Geometry check sheet. Reference: the model listing, model coordinates, mm. Face numbers are marked on the shaded views. A direction names the side the tool comes from. Round coordinates to 2 decimals unless told otherwise and drop trailing zeros. Order: outer loops, then holes, each group sorted by start corner. A loop starts at its lowest first (then second) coordinate and runs counter-clockwise, first axis right, second up. Notation, with made-up numbers: (60, 6) -> (110, 6) arc R24 cw to (110, 28) -> close; hole circle Ø10 at (69, 2.5). An arc over 180 degrees is marked (long way). Use a Markdown table: item, result. Add a question column.
Item 1: Gauge pin test, flat ends, axial feed: pin 1 Ø1 at (x, z) = (-2, 1) entering from -Y; pin 2 Ø1 at (x, z) = (2.5, 0) entering from +Y; pin 3 Ø3 at (x, y) = (-1.5, 2) entering from +Z. Record the tip position at first contact, or that the pin passes through.
Item 2: Sectioned sample at D-D, the plane x = -2.25. Record the cut outline in (y, z), and give its area (3 significant figures).
Item 3: Set-up check for the marked faces 4 and 5: record each of +Z, -Z, +X, -X, +Y, -Y from which the full face is reachable in a straight line by a thin tool's end or side.
Item 4: Material ranges on probe 1 along Y at (x, z) = (0, -1.95); probe 2 along Y at (x, z) = (0, 0.1); probe 3 along Z at (x, y) = (2.25, -2), recorded low to high. Write a range as [from, to].
Item 5: Sectioned sample at A-A, the plane x = 0. Record the cut outline in (y, z), and give its area (3 significant figures).
Item 6: Sectioned sample at C-C, the plane z = 0.25. Record the cut outline in (x, y), and give its area (3 significant figures).
Item 7: Mould release check, pull along X, two halves, no side actions. Record for the marked faces 1, 2 and 3: pulls with the +X half, pulls with the -X half, needs draft (parallel to the pull), parting line crosses it, or undercut.
Autodesk Inventor part; units mm, degrees
ref_plane "YZ Plane" through (0, 0, 0) normal (1, 0, 0) x (0, 1, 0)
ref_plane "XZ Plane" through (0, 0, 0) normal (0, 1, 0) x (-1, 0, 0)
ref_plane "XY Plane" through (0, 0, 0) normal (0, 0, 1) x (1, 0, 0)
sketch "スケッチ1" plane through (0, 0, 0) normal (0, 0, 1) x (1, 0, 0)
  circle A0 centre (0, 0) radius 1.5
  circle A1 centre (0, 0) radius 4
  circle A2 centre (0, 0) radius 2
  circle A3 centre (0, 0) radius 3.5
  dimension "d0" = 3
  dimension "d1" = 8
  dimension "d2" = 4
  dimension "d3" = 0.5
extrude "押し出し1" add sketch "スケッチ1" along normal blind 2 contours A1 | A2 | A3
extrude "押し出し2" cut sketch "スケッチ1" against normal blind 0.1 from surface at 2 contours A3
mirror "ミラー1" about plane through (0, 0, 0) normal (0, 0, -1) of "押し出し1", "押し出し2"
properties part number "693ZZ" material "ステンレス鋼"
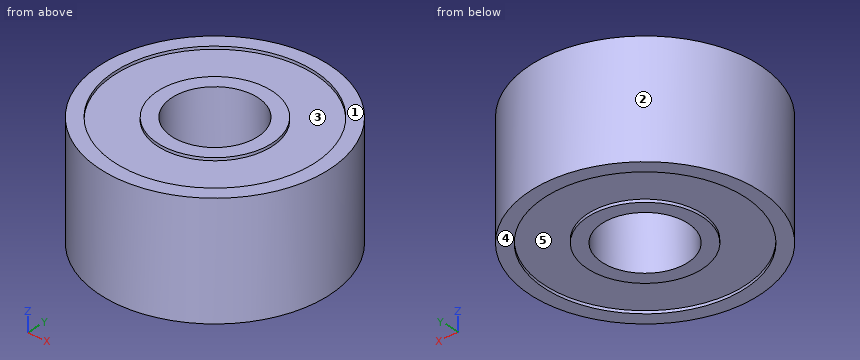
Found:
| question | item | result |
|---|---|---|
| 1 | pin 1 | stops at y = -3.71 |
| 1 | pin 2 | stops at y = 3.46 |
| 1 | pin 3 | stops at z = 2 |
| 2 | outline | (-3.31, -2) -> (-2.68, -2) -> (-2.68, -1.9) -> (2.68, -1.9) -> (2.68, -2) -> (3.31, -2) -> (3.31, 2) -> (2.68, 2) -> (2.68, 1.9) -> (-2.68, 1.9) -> (-2.68, 2) -> (-3.31, 2) -> close |
| 2 | area | 25.4 mm2 |
| 3 | face 4 | -Z, +X, -X, +Y, -Y |
| 3 | face 5 | -Z |
| 4 | probe 1 | y = [-4, -3.5], [-2, -1.5], [1.5, 2], [3.5, 4] |
| 4 | probe 2 | y = [-4, -1.5], [1.5, 4] |
| 4 | probe 3 | z = [-1.9, 1.9] |
| 5 | outline | (-4, -2) -> (-3.5, -2) -> (-3.5, -1.9) -> (-2, -1.9) -> (-2, -2) -> (-1.5, -2) -> (-1.5, 2) -> (-2, 2) -> (-2, 1.9) -> (-3.5, 1.9) -> (-3.5, 2) -> (-4, 2) -> close; (1.5, -2) -> (2, -2) -> (2, -1.9) -> (3.5, -1.9) -> (3.5, -2) -> (4, -2) -> (4, 2) -> (3.5, 2) -> (3.5, 1.9) -> (2, 1.9) -> (2, 2) -> (1.5, 2) -> close |
| 5 | area | 19.4 mm2 |
| 6 | outline | circle Ø8 at (0, 0); hole circle Ø3 at (0, 0) |
| 6 | area | 43.2 mm2 |
| 7 | face 1 | needs draft |
| 7 | face 2 | parting line crosses it |
| 7 | face 3 | undercut |
